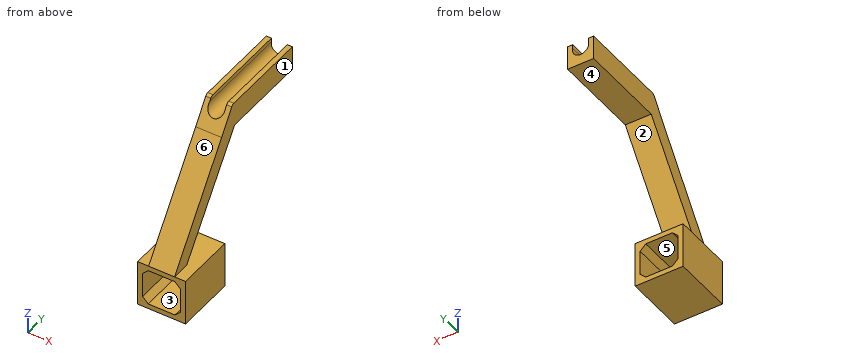
Autodesk Fusion 360 part; units mm, degrees
sketch "Sketch1" plane through (0, 0, 0) normal (0, 1, 0) x (1, 0, 0)
sketch "Sketch2" plane through (0, 0, 0) normal (1, 0, 0) x (0, 0, -1)
sketch "Sketch3" plane through (0, 0, 0) normal (0, 1, 0) x (1, 0, 0)
sketch "Sketch4" plane through (0, 0, 0) normal (0, 1, 0) x (1, 0, 0)
  line L0 (1.5, 7) -> (-5, 7)
  line L1 (8, -10) -> (10.5, -7.5)
  line L2 (10.5, -1.5) -> (10.5, -7.5)
  line L3 (-7.5, -1.5) -> (-7.5, -7.5)
  line L4 (1.5, 7) -> (8, 7)
  line L5 (10.5, -1.5) -> (10.5, -7.5)
  line L6 (1.5, -10) -> (8, -10)
  line L7 (10.5, -10) -> (-7.5, 7) construction
  line L8 (1.5, -10) -> (8, -10)
  line L9 (10.5, 7) -> (10.5, -10)
  line L10 (8, 7) -> (10.5, 4.5)
  line L11 (-7.5, -1.5) -> (-7.5, 4.5)
  line L12 (10.5, -1.5) -> (10.5, 4.5)
  line L13 (-7.5, 7) -> (10.5, 7)
  line L14 (-7.5, -7.5) -> (-5, -10)
  line L15 (-7.5, -10) -> (10.5, 7) construction
  line L16 (-7.5, 4.5) -> (-5, 7)
  line L17 (-7.5, -10) -> (-7.5, 7)
  line L18 (10.5, -10) -> (-7.5, -10)
  line L19 (1.5, -10) -> (-5, -10)
  line L20 (13.5, 10) -> (-10.5, 10)
  line L21 (-10.5, 10) -> (-10.5, -13)
  line L22 (-10.5, -13) -> (13.5, -13)
  line L23 (13.5, -13) -> (13.5, 10)
  line L24 (13.5, 10) -> (-10.5, -13) construction
  line L25 (-10.5, 10) -> (13.5, -13) construction
  line L26 (1.5, -10.5) -> (-5.2071, -10.5)
  line L27 (-8, -7.7071) -> (-5.2071, -10.5)
  line L28 (-8, -1.5) -> (-8, -7.7071)
  line L29 (-8, -1.5) -> (-8, 4.7071)
  line L30 (-8, 4.7071) -> (-5.2071, 7.5)
  line L31 (1.5, 7.5) -> (-5.2071, 7.5)
  line L32 (1.5, 7.5) -> (8.2071, 7.5)
  line L33 (8.2071, 7.5) -> (11, 4.7071)
  line L34 (11, -1.5) -> (11, 4.7071)
  line L35 (11, -1.5) -> (11, -7.7071)
  line L36 (8.2071, -10.5) -> (11, -7.7071)
  line L37 (1.5, -10.5) -> (8.2071, -10.5)
  point P0 (1.5, -1.5)
  point P1 (1.5, -1.5)
  point P2 (1.5, -1.5)
  dimension "d1" = 18
  dimension "d2" = 17
  dimension "d3" = 6
  dimension "d4" = 6
  dimension "d5" = 6.5
  dimension "d6" = 6.5
  dimension "d7" = 6
  dimension "d8" = 6
  dimension "d9" = 6.5
  dimension "d10" = 6.5
  dimension "d11" = 6.5
  dimension "d12" = 6
  dimension "d13" = 24
  dimension "d14" = 23
  dimension "d15" = -0.5
extrude "Extrude1" add sketch "Sketch4" along normal blind 30 contours L13 L17 L30 | L9 L13 L33 | L17 L18 L27 | L9 L18 L36 | L20 L21 L22 L23 makes body 1
sketch "Sketch5" plane through (0, 0, 0) normal (0, -1, 0) x (1, 0, 0)
  line L0 (-8, -4.7071) -> (-8, 7.7071)
  line L1 (-8, 7.7071) -> (-5.2071, 10.5)
  line L2 (-5.2071, 10.5) -> (8.2071, 10.5)
  line L3 (8.2071, 10.5) -> (11, 7.7071)
  line L4 (11, 7.7071) -> (11, -4.7071)
  line L5 (11, -4.7071) -> (8.2071, -7.5)
  line L6 (8.2071, -7.5) -> (-5.2071, -7.5)
  line L7 (-5.2071, -7.5) -> (-8, -4.7071)
  line L8 (13.5, -10) -> (13.5, 13)
  line L9 (13.5, 13) -> (-10.5, 13)
  line L10 (-10.5, 13) -> (-10.5, -10)
  line L11 (-10.5, -10) -> (13.5, -10)
  line L12 (-10.5, 13) -> (13.5, -10)
  line L13 (13.5, 13) -> (-10.5, -10)
  point P0 (1.5, 1.5)
sketch "Sketch6" plane through (0, 0, 0) normal (0, -1, 0) x (1, 0, 0)
  line L0 (-8, -4.7071) -> (-8, 7.7071)
  line L1 (-8, 7.7071) -> (-5.2071, 10.5)
  line L2 (-5.2071, 10.5) -> (8.2071, 10.5)
  line L3 (8.2071, 10.5) -> (11, 7.7071)
  line L4 (11, 7.7071) -> (11, -4.7071)
  line L5 (11, -4.7071) -> (8.2071, -7.5)
  line L6 (8.2071, -7.5) -> (-5.2071, -7.5)
  line L7 (-5.2071, -7.5) -> (-8, -4.7071)
  line L8 (13.5, -10) -> (13.5, 13)
  line L9 (13.5, 13) -> (-10.5, 13)
  line L10 (-10.5, 13) -> (-10.5, -10)
  line L11 (-10.5, -10) -> (13.5, -10)
  line L12 (1.5, 13) -> (1.5, 73)
  dimension "d18" = 60
ref_plane "WorkPlane1" through (1.5, 0, 43) normal (0, -1, 0) x (0, 0, 1)
sketch "Sketch7" plane through (1.5, 0, 43) normal (0, -1, 0) x (0, 0, 1)
  line L0 (-30, 0) -> (-30, -90)
  dimension "d20" = 90
ref_plane "WorkPlane2" through (46.5, 0, 13) normal (0, 0, -1) x (1, 0, 0)
sketch "Sketch25" plane through (1.5, 0, 43) normal (0, -1, 0) x (1, 0, 0)
  circle A0 centre (0, 30) radius 4.075
  dimension "d74" = 8.15
sketch "Sketch26" plane through (0, 0, 0) normal (0, 1, 0) x (1, 0, 0)
  circle A0 centre (1.5, -73) radius 4.075
  line L0 (8, -74) -> (-5, -74)
  line L1 (-5, -74) -> (-5, -63.85)
  line L2 (-5, -63.85) -> (8, -63.85)
  line L3 (8, -63.85) -> (8, -74)
  line L4 (8, -74) -> (-5, -63.85) construction
  line L5 (-5, -74) -> (8, -63.85) construction
  point P0 (1.5, -68.925)
extrude "Extrude18" add sketch "Sketch26" along normal blind 90 separate body contours A0 L0 L1 L2 L3 makes body 2
extrude "Extrude19" add 2 faces at (-3.3003, 60, 74) (7.1501, 30, 74) along direction (0, 0, 1) blind 2 on bodies 2 bodies 2
sketch "Sketch27" plane through (8, 0, 0) normal (1, 0, 0) x (0, 0, -1)
  line L0 (-76, 0) -> (-63.85, 0)
  line L1 (-63.85, 0) -> (-63.85, 90)
  line L2 (-63.85, 90) -> (-76, 90)
  line L3 (-76, 90) -> (-76, 0)
  line L4 (-13, 0) -> (10, 0)
  line L5 (10, 0) -> (10, 30)
  line L6 (10, 30) -> (-13, 30)
  line L7 (-13, 30) -> (-13, 0)
  line L8 (-63.85, 90) -> (-13, 30)
  line L9 (-63.85, 90) -> (-63.85, 75)
  line L10 (-13, 30) -> (-13, 15)
  line L11 (-63.85, 75.12) -> (-13, 15)
  line L12 (-63.85, 45) -> (-38.425, 45.06)
  line L13 (-63.85, 35.9416) -> (-30.7126, 35.9416)
  line L14 (-63.85, 35.9416) -> (-76, 35.9416)
extrude "Extrude20" cut sketch "Sketch27" against normal blind 30 contours L0 L1 L3 L14 bodies 2
sketch "Sketch32" plane through (-5, 0, 0) normal (-1, 0, 0) x (0, 0, 1)
  line L0 (63.85, 35.9416) -> (76, 35.9416)
  line L1 (76, 35.9416) -> (76, 90)
  line L2 (76, 90) -> (63.85, 90)
  line L3 (63.85, 90) -> (63.85, 35.9416)
  line L4 (-10, 0) -> (13, 0)
  line L5 (13, 0) -> (13, 30)
  line L6 (13, 30) -> (-10, 30)
  line L7 (-10, 30) -> (-10, 0)
  line L8 (63.85, 35.9416) -> (13, 0)
  line L9 (63.85, 35.9416) -> (63.85, 45.9416)
  line L10 (63.85, 45.9416) -> (13, 9.2584)
  dimension "d108" = 10
extrude "Extrude28" add sketch "Sketch32" against normal blind 13 contours L3 L5 L8 L9 L10 bodies 1 2
sketch "Sketch33" plane through (8, 0, 0) normal (1, 0, 0) x (0, 0, -1)
  line L0 (-63.85, 35.9416) -> (-83, 49)
  line L1 (-63.85, 35.9416) -> (-76, 35.9416)
  line L2 (-76, 90) -> (-76, 0)
  line L3 (-63.85, 35.9416) -> (-13, 0)
extrude "Extrude29" cut sketch "Sketch33" against normal blind 38 bodies 1
fillet "Fillet4" radius 2 2 edges at (-3.7252, 44.2267, 76) (6.7252, 44.2267, 76) on bodies 1
equation "d13 = 18.000 mm + 6 mm"
equation "d14 = 17.000 mm + 6 mm"
Read the model definition and answer for the solid it produces. Units are mm, in the model's axes. Face numbers are marked on the shaded views. A direction names the side the tool comes from. Round coordinates to 2 decimals unless told otherwise and drop trailing zeros. Write each loop counter-clockwise with the first axis right and the second up, starting at its lowest first coordinate (ties: lowest second). Pieces come first, ordered by that corner, then holes.
Q1. Find section B-B on y = 23.5. Determine the outline of the cut face in (x, z).
Values:
outline: (-10.5, -10) - (13.5, -10) - (13.5, 13) - (-10.5, 13) - close; (-5, 32.74) - (8, 32.74) - (8, 46.25) - (-5, 46.25) - close; hole (-8, -4.71) - (-5.21, -7.5) - (8.21, -7.5) - (11, -4.71) - (11, 7.71) - (8.21, 10.5) - (-5.21, 10.5) - (-8, 7.71) - close
Q2. Straight lines are drawn through the part: line 1 (X direction, y = 59, z = 73) (3 decimals); line 2 (X direction, y = 25.5, z = -2); line 3 (Z direction, x = 3.25, y = 29). For each, find the intervals that lie inside material, in ascending order.
Values:
line 1: x = -5 to -2.575, 5.575 to 8
line 2: x = -10.5 to -8, 11 to 13.5
line 3: z = -10 to -7.5, 10.5 to 13, 40.37 to 54.03
Q3. Find section C-C on y = 79. Determine the outline of the cut face in (x, z) (3 decimals), and give its area (3 significant figures).
Values:
outline: (-5, 63.85) - (8, 63.85) - (8, 76) - (5.45, 76) - (5.45, 74) arc R4.075 cw (long way) to (-2.45, 74) - (-2.45, 76) - (-5, 76) - close
area: 108 mm2
Q4. Find section D-D on z = 40. Determine the outline of the cut face in (x, y).
Values:
outline: (-5, 19.08) - (8, 19.08) - (8, 28.74) - (-5, 28.74) - close
Q5. Find section A-A on x = 1.5. Determine the outline of the cut face in (y, z) (3 decimals), and give its area (3 significant figures).
Values:
outline: (0, -10) - (30, -10) - (30, -7.5) - (0, -7.5) - close; (0, 10.5) - (30, 10.5) - (30, 13) - (9.258, 13) - (45.942, 63.85) - (90, 63.85) - (90, 68.925) - (39.402, 68.925) - (35.942, 63.85) - (0, 13) - close
area: 905 mm2
Q6. Flat-ended cylindrical pins translate along their axes: P1, Ø10, axis at x = 0.5, z = 6.5, coming from the +Y side; P2, Ø6.5, axis at x = -1, y = 18, coming from the +Z side; P3, Ø6, axis at x = 8.5, z = 7, coming from the -Y side; P4, Ø2, axis at x = 5, z = 25, coming from the -Y side (3 decimals). Find the tip coordinate at first contact, or state that the pin passes through.
Values:
P1: stops at y = 30
P2: stops at z = 43.06
P3: stops at y = 0
P4: stops at y = 7.775
Q7. A tool of negligible diameter and unlimited length cuts with its end or side. For the marked faces 4, 5 and 6, from which of +Z, -Z, +X, -X, +Y, -Y can it reach the whole face along a straight path? Write none if from no direction.
Values:
face 4: -Z, +X, -X, +Y
face 5: +Y, -Y
face 6: +Z, +X, -X, -Y
Q8. The mould has two halves that part along X. Classify the marked faces 1, 2 and 3: released by +X, released by -X, zero draft, split by the parting line, or undercut.
Values:
face 1: released by +X
face 2: zero draft
face 3: undercut
